```python
from build123d import *

# Parameters (mm, degrees)
SKETCH1_R           = 24.81
BOSS_EXTRUDE1_DEPTH = 12.96
SKETCH3_R           = 24.205
CUT_EXTRUDE2_DEPTH  = 11.25
SKETCH4_R           = 21.33
CUT_EXTRUDE3_DEPTH  = 11.25


with BuildPart() as part:
    # Sketch1 → Boss-Extrude1 (new body)
    with BuildSketch(Plane.XY):
        Circle(SKETCH1_R)
    extrude(amount=BOSS_EXTRUDE1_DEPTH)

    # Sketch3 → Cut-Extrude2 (cut)
    with BuildSketch(Plane(origin=(0, 0, 0), x_dir=(-1, 0, 0), z_dir=(0, 0, -1))):
        Circle(SKETCH3_R)
    extrude(amount=-CUT_EXTRUDE2_DEPTH, mode=Mode.SUBTRACT)

    # Sketch4 → Cut-Extrude3 (cut)
    with BuildSketch(Plane.XY.offset(12.96)):
        Circle(SKETCH4_R)
    extrude(amount=-CUT_EXTRUDE3_DEPTH, mode=Mode.SUBTRACT)


solid = part.part
```
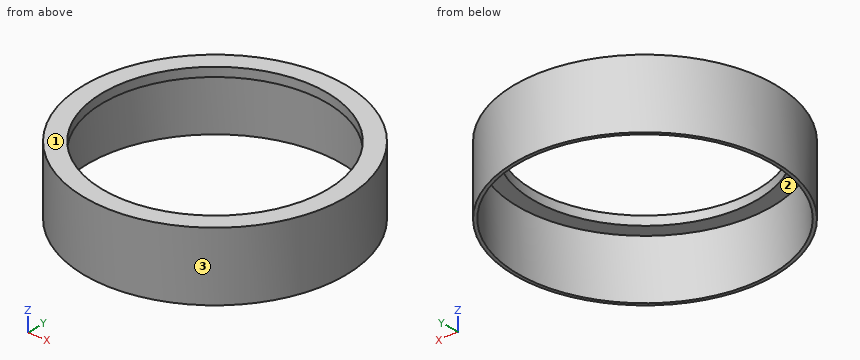
Source: CAD feature listing. Evaluate the final solid. Frame: model axes, mm. Face numbers are marked on the shaded views. Coordinates: 2 decimals unless noted, no trailing zeros. Loops run counter-clockwise (first coordinate to the right, second up) from the corner with the lowest first, then second, coordinate; pieces in that order, holes last. Notation, with made-up numbers: M -29.5,29.25 L 13.5,29.25 A27 ccw 13.5,48.25 Z; hole C -31.75,-14.75 d2. An arc over 180 degrees is marked long. Use CSV: the item, a comma, the result in double quotes.
(1) Draft query along X for the marked faces 1, 2 and 3. Return one class per face: pulls with the +X half, pulls with the -X half, needs draft (parallel to the pull), parting line crosses it, or undercut.
Answers follow:
face 1,"needs draft"
face 2,"undercut"
face 3,"parting line crosses it"
(2) Cut plane C-C on z = 7.25. Return loops of the section in (x, y) (3 decimals), and give its area (3 significant figures).
Answers follow:
outline,"C 0,0 d49.62; hole C 0,0 d48.41"
area,"93.2 mm²"
(3) Line query: line 1 (Y direction, x = 0, z = 4.5) (3 decimals); line 2 (Y direction, x = 0, z = 11.7); line 3 (X direction, y = -20, z = 4.25). Output: solid intervals per line, ascending. Write a range as [from, to].
Answers follow:
line 1,"[-24.81, -24.205], [24.205, 24.81]"
line 2,"[-24.81, -21.33], [21.33, 24.81]"
line 3,"[-14.68, -13.63], [13.63, 14.68]"
(4) Contact query for flat-ended pins moving along their axis: pin 1 (5 mm diameter, centred on x = -8, z = 10, fed in from -Y); pin 2 (4 mm diameter, centred on x = -5, z = 8, fed in from +Y); pin 3 (2 mm diameter, centred on y = 16, z = 5, fed in from -X). Output: stop coordinate, or through.
Answers follow:
pin 1,"y = -24.19"
pin 2,"y = 24.63"
pin 3,"x = -19.76"
(5) Cut plane A-A on x = 0. Return loops of the section in (y, z) (3 decimals).
Answers follow:
outline,"M -24.81,0 L -24.205,0 L -24.205,11.25 L -21.33,11.25 L -21.33,12.96 L -24.81,12.96 Z; M 21.33,11.25 L 24.205,11.25 L 24.205,0 L 24.81,0 L 24.81,12.96 L 21.33,12.96 Z"
